For this review, take the finished solid that the model builds, in its own axes (mm). Face numbers are marked on the shaded views. Coordinates: 2 decimals unless noted, no trailing zeros. Write each loop counter-clockwise with the first axis right and the second up, starting at its lowest first coordinate (ties: lowest second). Pieces come first, ordered by that corner, then holes.
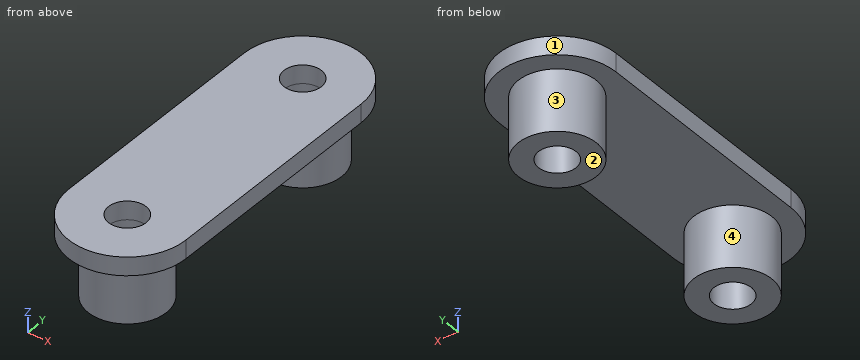
```python
from build123d import *

# Parameters (mm, degrees)
SKETCH1_R           = 1.524
BOSS_EXTRUDE1_DEPTH = 1.5
SKETCH1_7_R         = 3.175
SKETCH1_7_R_2       = 1.524
BOSS_EXTRUDE2_DEPTH = 5


with BuildPart() as part:
    # Sketch1 → Boss-Extrude1 (new body)
    with BuildSketch(Plane.XY):
        with BuildLine():
            Line((9.525, 0), (9.525, -19.05))
            ThreePointArc((9.525, -19.05), (4.7625, -23.8125), (0, -19.05))
            Line((0, -19.05), (0, 0))
            ThreePointArc((0, 0), (4.7625, 4.7625), (9.525, 0))
        make_face()
        with Locations((4.7625, 0)):
            Circle(SKETCH1_R, mode=Mode.SUBTRACT)
        with Locations((4.7625, -19.05)):
            Circle(SKETCH1_R, mode=Mode.SUBTRACT)
    extrude(amount=BOSS_EXTRUDE1_DEPTH)

    # Sketch1_7 → Boss-Extrude2 (add)
    with BuildSketch(Plane.XY):
        with Locations((4.7625, 0)):
            Circle(SKETCH1_7_R)
        with Locations((4.7625, 0)):
            Circle(SKETCH1_7_R_2, mode=Mode.SUBTRACT)
        with Locations((4.7625, -19.05)):
            Circle(SKETCH1_7_R)
        with Locations((4.7625, -19.05)):
            Circle(SKETCH1_7_R_2, mode=Mode.SUBTRACT)
    extrude(amount=-BOSS_EXTRUDE2_DEPTH)


solid = part.part
```
1) For L1, parallel to Y at x = 4, z = -0.25; L2, parallel to Y at x = 5, z = -1.75; L3, parallel to Y at x = 2, z = -2 (3 decimals), list the stretches that pass through material, from the lowest coordinate up.
2) Consider section B-B (x = 4.75). Give the boundary of the cut face in (y, z).
3) Clearance check with flat-ended pins moving along their axes: P1, Ø3, axis at x = 4, y = -8, coming from the -Z side; P2, Ø4, axis at x = 4.76, y = -19.05, coming from the +Z side; P3, Ø1.8, axis at x = 4.76, y = 0, coming from the -Z side; P4, Ø1, axis at x = 2.5, z = -2.5, coming from the +Y side. State where each tip first meets the part, or that it passes through.
4) Consider section C-C (y = 2.75). Give the boundary of the cut face in (x, z), then the cut area to 3 significant figures.
5) Consider section D-D (x = 8.5). Give the boundary of the cut face in (y, z).
6) Consider section A-A (z = 0.25). Count the separate pieces of the cut face and the enclosed holes in it, then the cut area to 3 significant figures.
7) The part is to be moulded in two halves that separate along Y. For the marked faces 1, 2, 3 and 4, say which applies: pulls with the +Y half, pulls with the -Y half, needs draft (parallel to the pull), parting line crosses it, or undercut.
Results:
1. L1: y = -22.13 to -20.37, -17.73 to -15.97, -3.08 to -1.32, 1.32 to 3.08
1. L2: y = -22.22 to -20.56, -17.54 to -15.88, -3.17 to -1.51, 1.51 to 3.17
1. L3: y = -20.615 to -17.485, -1.565 to 1.565
2. outline: (-23.81, 0) - (-22.22, 0) - (-22.22, -5) - (-20.57, -5) - (-20.57, 1.5) - (-23.81, 1.5) - close; (-17.53, -5) - (-15.88, -5) - (-15.88, 0) - (-3.17, 0) - (-3.17, -5) - (-1.52, -5) - (-1.52, 1.5) - (-17.53, 1.5) - close; (1.52, -5) - (3.17, -5) - (3.17, 0) - (4.76, 0) - (4.76, 1.5) - (1.52, 1.5) - close
3. P1: stops at z = 0
3. P2: stops at z = 1.5
3. P3: passes through
3. P4: stops at y = 2.64
4. outline: (0.87, 0) - (3.18, 0) - (3.18, -5) - (6.35, -5) - (6.35, 0) - (8.65, 0) - (8.65, 1.5) - (0.87, 1.5) - close
4. area: 27.5 mm2
5. outline: (-22, 0) - (2.95, 0) - (2.95, 1.5) - (-22, 1.5) - close
6. separate pieces: 1
6. enclosed holes: 2
6. area: 238 mm2
7. face 1: pulls with the +Y half
7. face 2: needs draft
7. face 3: undercut
7. face 4: undercut
